Could you check a few things on this model? Use its own coordinates, in mm. A direction names the side the tool comes from. Give positions to 0.01 mm unless a question says otherwise; leave off trailing zeros. Loops run counter-clockwise (first coordinate to the right, second up) from the corner with the lowest first, then second, coordinate; pieces in that order, holes last. Notation, with made-up numbers: (-32.5, 75) - (-22.5, 75) arc R24 ccw to (-22.5, 94) - close; hole circle Ø9 at (73.5, 17.5). An arc over 180 degrees is marked (long way). Write each question's results on one line, items separated by ' | '. Start each with the question number.
(1) For pin 1 (1 mm diameter, centred on y = 0.5, z = -51.5, fed in from +X); pin 2 (1.5 mm diameter, centred on y = 2, z = -11.5, fed in from +X); pin 3 (1.5 mm diameter, centred on y = 1, z = -83.5, fed in from +X), each with a flat end and sliding along its axis, tell me the tip position at first contact or that it passes through.
(2) I need wall thicknesses on line 1 (Z direction, x = 18, y = 1.1); line 2 (Z direction, x = 21, y = 1.8); line 3 (Y direction, x = 11, z = -31). Which ranges of each line are inside material? Lowest first, please.
(3) Suppose I cut it at A-A (y = 2.2). Please give me the cut outline in (x, z).
(4) Suppose I cut it at B-B (x = 36). Please give me the cut outline in (y, z).
(5) If we mould it in two halves opening along Z, with no side actions, what happens to faces 3 (the face through (36, 1, -95.5)), 4 (the face through (21.48, 1.48, -48.1)), 5 (the face through (35, 2, -95)), 6 (the face through (17.9, 3, -40.5))? For each: released by +Z, released by -Z, zero draft, split by the parting line, or undercut.
(6) On a 3-axis mill with a long thin cutter (end or side, diameter ignored), from which of +Z, -Z, +X, -X, +Y, -Y can I reach the whole of each face in a straight line? I mean faces 1 (the face through (11.7, 1.5, -55.7)), 2 (the face through (16, 1, -51)). Say none if no direction works.
from build123d import *

# Parameters (mm, degrees)
EXTRUDE_1_DEPTH      = 1
EXTRUDE_2_DEPTH      = 2
EXTRUDE_2_DEPTH_BACK = 1
EXTRUDE_4_DEPTH      = 2
EXTRUDE_4_DEPTH_BACK = 1
EXTRUDE_5_DEPTH      = 2


with BuildPart() as part:
    # Sketch 1 → Extrude 1 (new body)
    with BuildSketch(Plane(origin=(0, 0, 0), x_dir=(1, 0, 0), z_dir=(0, 1, 0))):
        Polygon((0, 0), (-5.8291827, 14.170729157), (29.567552432, 95.5), (41.564226141, 95.5), align=None)
    extrude(amount=EXTRUDE_1_DEPTH)



with BuildPart() as body_2:
    # Sketch 2 → Extrude 2 (new, two sides: drawn at the far end of the back side and taken through both)
    with BuildSketch(Plane(origin=(0, 1, 0), x_dir=(1, 0, 0), z_dir=(0, 1, 0)).offset(-EXTRUDE_2_DEPTH_BACK)):
        Polygon((0, 0), (41.564226141, 95.5), (42.109529491, 95.5), (0.26496285, -0.644124053), align=None)
    extrude(amount=EXTRUDE_2_DEPTH + EXTRUDE_2_DEPTH_BACK)


with BuildPart() as part_1:
    add(part.part)

    add(body_2.part)  # Extrude 4 merges body 2
    # Sketch 2_4 → Extrude 4 (add, two sides: drawn at the far end of the back side and taken through both)
    with BuildSketch(Plane(origin=(0, 1, 0), x_dir=(1, 0, 0), z_dir=(0, 1, 0)).offset(-EXTRUDE_4_DEPTH_BACK)):
        Polygon((-5.8291827, 14.170729157), (29.567552432, 95.5), (29.022249082, 95.5), (-6.09414555, 14.81485321), align=None)
    extrude(amount=EXTRUDE_4_DEPTH + EXTRUDE_4_DEPTH_BACK)

    # Sketch 7 → Extrude 5 (add)
    with BuildSketch(Plane(origin=(0, 1, 0), x_dir=(1, 0, 0), z_dir=(0, 1, 0))):
        Polygon((41.564226141, 95.5), (29.567552432, 95.5), (29.349938683, 95), (41.346612391, 95), align=None)
    extrude(amount=EXTRUDE_5_DEPTH)


solid = part_1.part
Output values:
1) pin 1: x = 23.18 | pin 2: x = 5.88 | pin 3: x = 37.21
2) line 1: -70.17 to -68.92, -41.36 to -40.1 | line 2: -77.07 to -75.81, -48.25 to -47 | line 3: 0 to 1
3) outline: (-6.09, -14.81) - (29.02, -95.5) - (42.11, -95.5) - (0.26, 0.64) - (0, 0) - (41.35, -95) - (29.35, -95) - (-5.83, -14.17) - close
4) outline: (0, -95.5) - (3, -95.5) - (3, -95) - (1, -95) - (1, -82.72) - (3, -82.72) - (3, -81.46) - (0, -81.46) - close
5) face 3: released by -Z | face 4: released by +Z | face 5: undercut | face 6: zero draft
6) face 1: -Z, -X, +Y, -Y | face 2: +Y
